Work out the finished part from the listing and answer in its coordinate system (mm). A direction names the side the tool comes from. Coordinates: 2 decimals unless noted, no trailing zeros. Order: outer loops, then holes, each group sorted by start corner. A loop starts at its lowest first (then second) coordinate and runs counter-clockwise, first axis right, second up. Notation, with made-up numbers: (55.25, -6.5) -> (75.25, -6.5) arc R17 cw to (75.25, 3.5) -> close; hole circle Ø5 at (19, -36.5). An arc over 180 degrees is marked (long way). Write item = value, one per line. Start each with the question number.
Q1. Straight lines are drawn through the part: L1, parallel to X at y = 75, z = 5.5; L2, parallel to Y at x = -82, z = 9.75; L3, parallel to X at y = 71.75, z = 8. For each, find the intervals that lie inside material, in ascending order. Write a range as from..to.
Q2. The part is cut by section B-B, the plane z = 1.75. Count the separate pieces of the cut face and the enclosed holes in it, plus the area to 3 significant figures.
Q3. The part is cut by section A-A, the plane x = -85.5. Determine the outline of the cut face in (y, z).
Q4. Which of the six approach directions +Z, -Z, +X, -X, +Y, -Y give full straight-line access (tool end or side, diameter ignored) to faces 4 (the flat face through (-100, 73, 10)), 5 (the flat face through (-59, 70.696, 5))?
Q5. For a pull along Y with two mould halves and no side action, classify faces 1 (the flat face through (-155.543, 73, 5)), 2 (the cylindrical face through (-75.21, 72.5, 4.93)), 3 (the flat face through (-100, 79.196, 5)) as +Y half, -Y half, draft (parallel to the pull), parting line (faces both ways), or undercut.
```python
from build123d import *

# Parameters (mm, degrees)
SKETCH1_W           = 112.520086359
SKETCH1_H           = 12
SKETCH1_R           = 2.5
SKETCH1_R_2         = 1.143
BOSS_EXTRUDE1_DEPTH = 10


with BuildPart() as part:
    # Sketch1 → Boss-Extrude1 (new body)
    with BuildSketch(Plane.XY):
        with Locations((-99.282747956, 73.19632446)):
            Rectangle(SKETCH1_W, SKETCH1_H)
        with Locations((-149.542791135, 73.19632446)):
            Circle(SKETCH1_R, mode=Mode.SUBTRACT)
        with Locations((-129.542791135, 73.19632446)):
            Circle(SKETCH1_R, mode=Mode.SUBTRACT)
        with Locations((-89.542791135, 73.19632446)):
            Circle(SKETCH1_R_2, mode=Mode.SUBTRACT)
        with Locations((-74.302791135, 73.19632446)):
            Circle(SKETCH1_R_2, mode=Mode.SUBTRACT)
        with Locations((-66.682791135, 73.19632446)):
            Circle(SKETCH1_R_2, mode=Mode.SUBTRACT)
        with Locations((-51.442791135, 73.19632446)):
            Circle(SKETCH1_R_2, mode=Mode.SUBTRACT)
        with BuildLine():
            Line((-84.422791135, 75.69632446), (-79.422791135, 75.69632446))
            ThreePointArc((-79.422791135, 75.69632446), (-76.922791135, 73.19632446), (-79.422791135, 70.69632446))
            Line((-79.422791135, 70.69632446), (-84.422791135, 70.69632446))
            ThreePointArc((-84.422791135, 70.69632446), (-86.922791135, 73.19632446), (-84.422791135, 75.69632446))
        make_face(mode=Mode.SUBTRACT)
        with BuildLine():
            Line((-61.562791135, 75.69632446), (-56.562791135, 75.69632446))
            ThreePointArc((-56.562791135, 75.69632446), (-54.062791135, 73.19632446), (-56.562791135, 70.69632446))
            Line((-56.562791135, 70.69632446), (-61.562791135, 70.69632446))
            ThreePointArc((-61.562791135, 70.69632446), (-64.062791135, 73.19632446), (-61.562791135, 75.69632446))
        make_face(mode=Mode.SUBTRACT)
    extrude(amount=BOSS_EXTRUDE1_DEPTH)


solid = part.part
```
Model answer:
q1.L1 = -155.54..-151.27, -147.81..-131.27, -127.81..-86.15, -77.69..-63.29, -54.83..-43.02
q1.L2 = 67.2..70.7, 75.7..79.2
q1.L3 = -155.54..-151.58, -147.5..-131.58, -127.5..-86.46, -77.38..-63.6, -54.52..-43.02
q2.separate_pieces = 1
q2.enclosed_holes = 8
q2.area = 1,210 mm2
q3.outline = (67.2, 0) -> (70.94, 0) -> (70.94, 10) -> (67.2, 10) -> close; (75.45, 0) -> (79.2, 0) -> (79.2, 10) -> (75.45, 10) -> close
q4.face_4 = +Z, +X, -X, +Y, -Y
q4.face_5 = +Z, -Z
q5.face_1 = draft
q5.face_2 = undercut
q5.face_3 = +Y half
